```python
from build123d import *

# Parameters (mm, degrees)
F0_W     = 29
F0_H     = 75
F0_R     = 1.8
F1_DEPTH = 5
F3_DEPTH = 29
F4_DEPTH = 2


with BuildPart() as f1:
    # F0 (on Top) → F1 (new body)
    with BuildSketch(Plane.XY):
        with Locations((14.5, -37.5)):
            Rectangle(F0_W, F0_H)
        Polygon((1.709103, -71.5), (3.354552, -68.65), (6.645448, -68.65), (8.290897, -71.5), (6.645448, -74.35), (3.354552, -74.35), align=None, mode=Mode.SUBTRACT)
        Polygon((20.709103, -71.5), (22.354552, -68.65), (25.645448, -68.65), (27.290897, -71.5), (25.645448, -74.35), (22.354552, -74.35), align=None, mode=Mode.SUBTRACT)
        with BuildLine():
            Line((5.85, -55), (5.85, -10))
            ThreePointArc((5.85, -10), (8, -7.85), (10.15, -10))
            Line((10.15, -10), (10.15, -55))
            ThreePointArc((10.15, -55), (8, -57.15), (5.85, -55))
        make_face(mode=Mode.SUBTRACT)
        with BuildLine():
            Line((18.85, -55), (18.85, -10))
            ThreePointArc((18.85, -10), (21, -7.85), (23.15, -10))
            Line((23.15, -10), (23.15, -55))
            ThreePointArc((23.15, -55), (21, -57.15), (18.85, -55))
        make_face(mode=Mode.SUBTRACT)
        Polygon((25.645448, -68.65), (22.354552, -68.65), (20.709103, -71.5), (22.354552, -74.35), (25.645448, -74.35), (27.290897, -71.5), align=None)
        with Locations((24, -71.5)):
            Circle(F0_R, mode=Mode.SUBTRACT)
        Polygon((6.645448, -68.65), (3.354552, -68.65), (1.709103, -71.5), (3.354552, -74.35), (6.645448, -74.35), (8.290897, -71.5), align=None)
        with Locations((5, -71.5)):
            Circle(F0_R, mode=Mode.SUBTRACT)
    extrude(amount=F1_DEPTH)

    # F2 (on face) → F3 (cut, through all)
    with BuildSketch(Plane.YZ.offset(29)):
        with BuildLine():
            Line((-64.5, 5), (-67.5, 5))
            ThreePointArc((-67.5, 5), (-66, 3.5), (-64.5, 5))
        make_face()
    extrude(amount=-F3_DEPTH, mode=Mode.SUBTRACT)

    # F0 (on Top) → F4 (cut)
    with BuildSketch(Plane.XY):
        with Locations((5, -71.5)):
            Circle(F0_R)
        with Locations((24, -71.5)):
            Circle(F0_R)
        Polygon((6.645448, -68.65), (3.354552, -68.65), (1.709103, -71.5), (3.354552, -74.35), (6.645448, -74.35), (8.290897, -71.5), align=None)
        with Locations((5, -71.5)):
            Circle(F0_R, mode=Mode.SUBTRACT)
        Polygon((25.645448, -68.65), (22.354552, -68.65), (20.709103, -71.5), (22.354552, -74.35), (25.645448, -74.35), (27.290897, -71.5), align=None)
        with Locations((24, -71.5)):
            Circle(F0_R, mode=Mode.SUBTRACT)
    extrude(amount=F4_DEPTH, mode=Mode.SUBTRACT)


solid = f1.part
```
Can you work these out from the model? Positions are in its coordinate system, mm. A direction names the side the tool comes from. Give positions to 0.01 mm unless a question says otherwise; leave off trailing zeros. Order: outer loops, then holes, each group sorted by start corner. A loop starts at its lowest first (then second) coordinate and runs counter-clockwise, first axis right, second up. Notation, with made-up numbers: M -34.75,63 L -6.75,63 A20 ccw -6.75,97 Z; hole C 78.5,25.5 d1. An arc over 180 degrees is marked long. One line per item, written item: value.
1) I want a section at B-B, the plane x = 24. List the corners of the cut face in (y, z) for me, plus the area to 3 significant figures.
Answer sheet:
outline: M -75,0 L -74.35,0 L -74.35,2 L -73.3,2 L -73.3,5 L -75,5 Z; M -69.7,2 L -68.65,2 L -68.65,0 L 0,0 L 0,5 L -64.5,5 A1.5 cw -67.5,5 L -69.7,5 Z
area: 349 mm^2
2) We'd pull the mould along X, two halves only. Please class faces 4 (the face through (14, 0, 2)), 5 (the face through (18.85, -33, 2)), 6 (the face through (0, -38, 2)), 7 (the face through (5.968, -69.982, 3.479)): released by +X, released by -X, zero draft, split by the parting line, or undercut.
Answer sheet:
face 4: zero draft
face 5: undercut
face 6: released by -X
face 7: undercut
3) I want a section at D-D, the plane y = -66. List the corners of the cut face in (x, z) for me, plus the area to 4 significant figures.
Answer sheet:
outline: M 0,0 L 29,0 L 29,3.5 L 0,3.5 Z
area: 101.5 mm^2
4) On a 3-axis mill with a long thin cutter (end or side, diameter ignored), from which of +Z, -Z, +X, -X, +Y, -Y can I reach the whole of each face in a straight line? I mean faces 1 (the face through (14, -71, 5)), 2 (the face through (10.15, -32, 2)), 3 (the face through (2.54, -70.06, 0.99)). Say none if no direction works.
Answer sheet:
face 1: +Z, +X, -X, +Y, -Y
face 2: +Z, -Z
face 3: -Z
5) For P1, Ø1.6, axis at x = 23.5, z = 1.5, coming from the +Y side; P2, Ø2, axis at x = 24, y = -71.5, coming from the +Z side; P3, Ø4.5, axis at x = 5, y = -71, coming from the -Z side, each with a flat end and sliding along its axis, tell me the tip position at first contact or that it passes through.
Answer sheet:
P1: stops at y = 0
P2: passes through
P3: stops at z = 2
6) Please list where these lines run through material, in increasing order: line 1 along X through (y, z) = (-36.5, 4.65); line 2 along X through (y, z) = (-71.5, 4.25); line 3 along Y through (x, z) = (5, 4.3).
Answer sheet:
line 1: x = 0 to 5.85, 10.15 to 18.85, 23.15 to 29
line 2: x = 0 to 3.2, 6.8 to 22.2, 25.8 to 29
line 3: y = -75 to -73.3, -69.7 to -67.33, -64.67 to 0
7) I want a section at C-C, the plane z = 4.2. List the corners of the cut face in (x, y) for me.
Answer sheet:
outline: M 0,-75 L 29,-75 L 29,-67.27 L 0,-67.27 Z; M 0,-64.73 L 29,-64.73 L 29,0 L 0,0 Z; hole C 5,-71.5 d3.6; hole M 5.85,-55 A2.15 ccw 10.15,-55 L 10.15,-10 A2.15 ccw 5.85,-10 Z; hole M 18.85,-55 A2.15 ccw 23.15,-55 L 23.15,-10 A2.15 ccw 18.85,-10 Z; hole C 24,-71.5 d3.6
8) I want a section at A-A, the plane y = -22. List the corners of the cut face in (x, z) for me.
Answer sheet:
outline: M 0,0 L 5.85,0 L 5.85,5 L 0,5 Z; M 10.15,0 L 18.85,0 L 18.85,5 L 10.15,5 Z; M 23.15,0 L 29,0 L 29,5 L 23.15,5 Z
